The drawing under review shows one solid part. Ordinate dimensions are in mm from its lowest x, y, z. A direction names the side the tool comes from. Coordinates: 2 decimals unless noted, no trailing zeros. Write each loop counter-clockwise with the first axis right and the second up, starting at its lowest first coordinate (ties: lowest second). Pieces come first, ordered by that corner, then holes. Notation, with made-up numbers: (36.5, 30) - (55.5, 30) arc R16 ccw to (55.5, 48) - close; hole circle Ø11 at (39, 2.5). An arc over 180 degrees is marked (long way). Use a Markdown table: item, result.
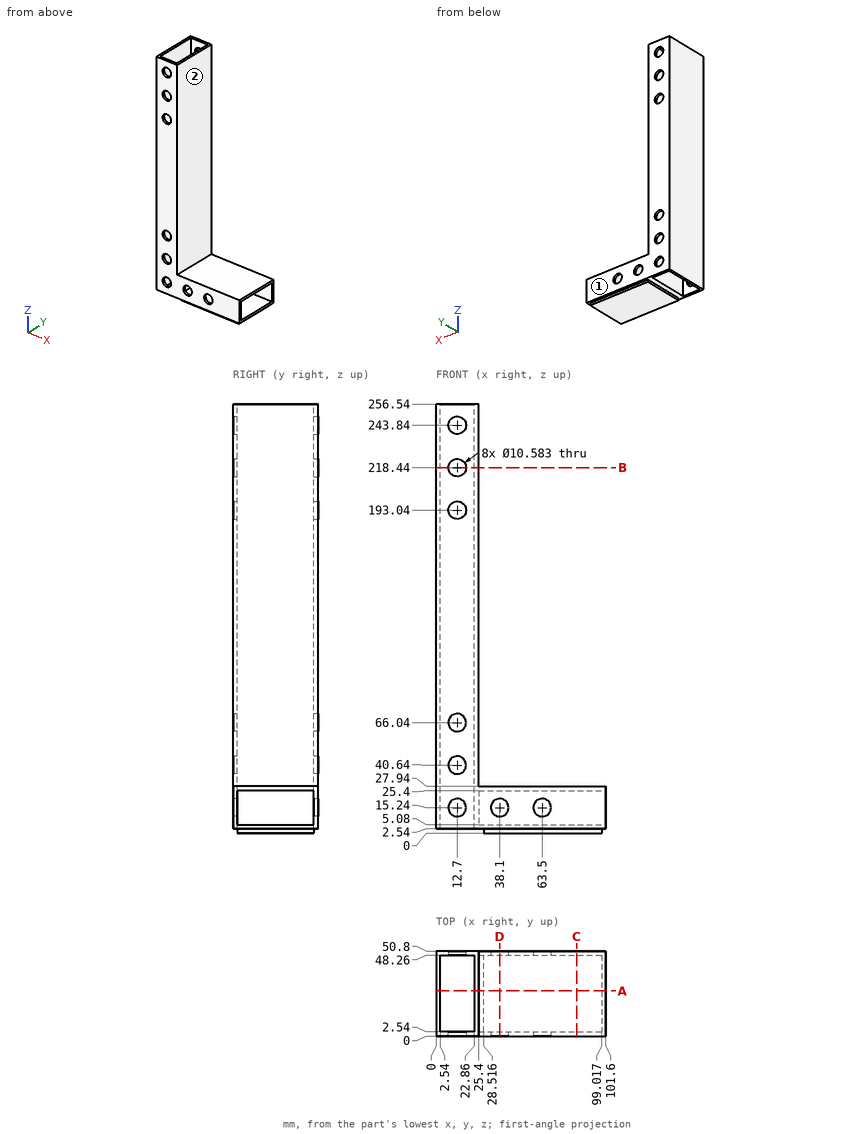
(1) Take a section at A-A on y = 27. Write out the cut boundary in (x, z), and give its area (3 significant figures).
Determined:
| item | result |
|---|---|
| outline | (0, 2.54) - (2.54, 2.54) - (2.54, 256.54) - (0, 256.54) - close; (22.86, 2.54) - (28.52, 2.54) - (28.52, 0) - (99.02, 0) - (99.02, 2.54) - (101.6, 2.54) - (101.6, 5.08) - (25.4, 5.08) - (25.4, 25.4) - (101.6, 25.4) - (101.6, 27.94) - (25.4, 27.94) - (25.4, 256.54) - (22.86, 256.54) - close |
| area | 1,860 mm2 |
(2) Take a section at C-C on x = 84. Write out the cut boundary in (y, z).
Determined:
| item | result |
|---|---|
| outline | (0, 2.54) - (2.54, 2.54) - (2.54, 0) - (48.26, 0) - (48.26, 2.54) - (50.8, 2.54) - (50.8, 27.94) - (0, 27.94) - close; hole (2.54, 5.08) - (48.26, 5.08) - (48.26, 25.4) - (2.54, 25.4) - close |
(3) Take a section at B-B on z = 218.44. Write out the cut boundary in (x, y).
Determined:
| item | result |
|---|---|
| outline | (0, 0) - (7.41, 0) - (7.41, 2.54) - (2.54, 2.54) - (2.54, 48.26) - (7.41, 48.26) - (7.41, 50.8) - (0, 50.8) - close; (17.99, 0) - (25.4, 0) - (25.4, 50.8) - (17.99, 50.8) - (17.99, 48.26) - (22.86, 48.26) - (22.86, 2.54) - (17.99, 2.54) - close |
(4) Machinability: for the marked faces 1 and 2, which of the approach directions +Z, -Z, +X, -X, +Y, -Y give a long, thin tool a straight path to every point of the face, cutting with its end or side? Answer none if there is none.
Determined:
| item | result |
|---|---|
| face 1 | +Z, -Z, +X, -X, +Y |
| face 2 | +Z, +X, +Y, -Y |
(5) Take a section at D-D on x = 38.1. Write out the cut boundary in (y, z).
Determined:
| item | result |
|---|---|
| outline | (0, 2.54) - (2.54, 2.54) - (2.54, 0) - (48.26, 0) - (48.26, 2.54) - (50.8, 2.54) - (50.8, 9.95) - (48.26, 9.95) - (48.26, 5.08) - (2.54, 5.08) - (2.54, 9.95) - (0, 9.95) - close; (0, 20.53) - (2.54, 20.53) - (2.54, 25.4) - (48.26, 25.4) - (48.26, 20.53) - (50.8, 20.53) - (50.8, 27.94) - (0, 27.94) - close |
(6) For pin 1 (8.5 mm diameter, centred on x = 12.7, z = 193.04, fed in from +Y); pin 2 (6 mm diameter, centred on x = 45.5, y = 22, fed in from +Z); pin 3 (23 mm diameter, centred on y = 16, z = 96.5, fed in from +X); pin 4 (1.3 mm diameter, centred on y = 36, z = 1, fed in from -X), all flat-tipped, find the tip position at first contact; note any pin that passes through.
Determined:
| item | result |
|---|---|
| pin 1 | through |
| pin 2 | z = 27.94 |
| pin 3 | x = 25.4 |
| pin 4 | x = 28.52 |
(7) For L1, parallel to X at y = 49, z = 15; L2, parallel to X at y = 47, z = 89.5; L3, parallel to Y at x = 5, z = 60, list the stretches that pass through material, from the lowest coordinate up. Write a range as from..to.
Determined:
| item | result |
|---|---|
| L1 | 0..7.41, 17.99..32.81, 43.39..58.21, 68.79..101.6 |
| L2 | 0..2.54, 22.86..25.4 |
| L3 | 0..2.54, 48.26..50.8 |
